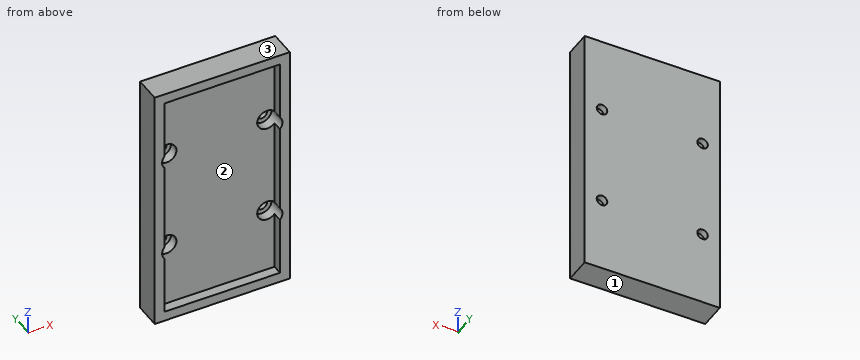
from build123d import *

# Parameters (mm, degrees)
SKETCH1_W                  = 35
SKETCH1_H                  = 70
BOSS_EXTRUDE1_DEPTH        = 5
EXTRUDE_THIN1_DEPTH        = 5
EXTRUDE_THIN1_DEPTH_BACK   = 3
SKETCH9_W                  = 41
SKETCH9_H                  = 76
SKETCH9_W_2                = 35
SKETCH9_H_2                = 70
F_3_2_3_2_DIAMETER_HOLE1_D = 3.2
CUT_EXTRUDE1_DEPTH         = 44.465503563
CUT_EXTRUDE1_DEPTH_BACK    = 3
SKETCH8_R                  = 3


with BuildPart() as part:
    # Sketch1 → Boss-Extrude1 (new body)
    with BuildSketch(Plane(origin=(0, 0, 0), x_dir=(1, 0, 0), z_dir=(0, 1, 0))):
        Rectangle(SKETCH1_W, SKETCH1_H)
    extrude(amount=-BOSS_EXTRUDE1_DEPTH)

    # Sketch9 → Extrude-Thin1 (add, two sides: drawn at the far end of the back side and taken through both)
    with BuildSketch(Plane(origin=(0, -5, 0), x_dir=(1, 0, 0), z_dir=(0, 1, 0)).offset(-EXTRUDE_THIN1_DEPTH_BACK)):
        Rectangle(SKETCH9_W, SKETCH9_H)
        Rectangle(SKETCH9_W_2, SKETCH9_H_2, mode=Mode.SUBTRACT)
    extrude(amount=EXTRUDE_THIN1_DEPTH + EXTRUDE_THIN1_DEPTH_BACK)

    # Ø3.2 (3.2) Diameter Hole1 (through all)
    with Locations(Plane(origin=(0, -5, 0), x_dir=(-1, 0, 0), z_dir=(0, -1, 0))):
        with Locations((15.25, 15.25), (15.25, -15.25), (-15.25, -15.25), (-15.25, 15.25)):
            Hole(F_3_2_3_2_DIAMETER_HOLE1_D / 2)

    # Sketch8 → Cut-Extrude1 (cut, two sides: drawn at the far end of the back side and taken through both)
    with BuildSketch(Plane.XZ.offset(5).offset(-CUT_EXTRUDE1_DEPTH_BACK)):
        with Locations(Location((-15.25, 15.25, 0), (0, 0, 138.590377891))):
            Circle(SKETCH8_R)
        with Locations(Location((15.25, 15.25, 0), (0, 0, 41.409622109))):
            Circle(SKETCH8_R)
        with Locations(Location((15.25, -15.25, 0), (0, 0, 41.409622109))):
            Circle(SKETCH8_R)
        with Locations(Location((-15.25, -15.25, 0), (0, 0, 138.590377891))):
            Circle(SKETCH8_R)
    extrude(amount=CUT_EXTRUDE1_DEPTH + CUT_EXTRUDE1_DEPTH_BACK, mode=Mode.SUBTRACT)


solid = part.part
Geometry check sheet. Reference: the model listing, model coordinates, mm. Face numbers are marked on the shaded views. Round coordinates to 2 decimals unless told otherwise and drop trailing zeros. Loops run counter-clockwise (first coordinate to the right, second up) from the corner with the lowest first, then second, coordinate; pieces in that order, holes last.
Item 1: Cross-section at C-C on y = -3.25. Record the boundary of the cut face in (x, z).
Item 2: Gauge pin test, flat end, axial feed: pin 1 (3.5 mm diameter, centred on x = -15.25, z = -15.25, fed in from -Y). Record the tip position at first contact, or that the pin passes through.
Item 3: Mould release check, pull along Z, two halves, no side actions. Record for the marked faces 1, 2 and 3: pulls with the +Z half, pulls with the -Z half, needs draft (parallel to the pull), parting line crosses it, or undercut.
Item 4: Cross-section at B-B on z = 15.25. Record the boundary of the cut face in (x, y), then the cut area to 3 significant figures.
Item 5: Thickness scan on line 1 (Z direction, x = -15.25, y = -1.2); line 2 (Z direction, x = -17.5, y = -2.25); line 3 (Z direction, x = -6, y = -7). Record the ranges inside material, lowest first.
Item 6: Cross-section at A-A on x = 15.25. Record the boundary of the cut face in (y, z), then the cut area to 3 significant figures.
Item 7: Cross-section at D-D on x = 6. Record the boundary of the cut face in (y, z).
Answer sheet:
1. outline: (-20.5, -38) - (20.5, -38) - (20.5, 38) - (-20.5, 38) - close; hole circle Ø6 at (-15.25, -15.25); hole circle Ø6 at (-15.25, 15.25); hole circle Ø6 at (15.25, -15.25); hole circle Ø6 at (15.25, 15.25)
2. pin 1: stops at y = -2
3. face 1: pulls with the -Z half
3. face 2: undercut
3. face 3: pulls with the +Z half
4. outline: (-20.5, -8) - (-18.25, -8) - (-18.25, -2) - (-16.85, -2) - (-16.85, 0) - (-20.5, 0) - close; (-13.65, -2) - (-12.25, -2) - (-12.25, -5) - (12.25, -5) - (12.25, -2) - (13.65, -2) - (13.65, 0) - (-13.65, 0) - close; (16.85, -2) - (18.25, -2) - (18.25, -8) - (20.5, -8) - (20.5, 0) - (16.85, 0) - close
4. area: 170 mm2
5. line 1: z = -38 to -16.85, -13.65 to 13.65, 16.85 to 38
5. line 2: z = -38 to -17.23, -13.27 to 13.27, 17.23 to 38
5. line 3: z = -38 to -35, 35 to 38
6. outline: (-8, -38) - (0, -38) - (0, -16.85) - (-2, -16.85) - (-2, -18.25) - (-5, -18.25) - (-5, -35) - (-8, -35) - close; (-8, 35) - (-5, 35) - (-5, 18.25) - (-2, 18.25) - (-2, 16.85) - (0, 16.85) - (0, 38) - (-8, 38) - close; (-5, -12.25) - (-2, -12.25) - (-2, -13.65) - (0, -13.65) - (0, 13.65) - (-2, 13.65) - (-2, 12.25) - (-5, 12.25) - close
6. area: 349 mm2
7. outline: (-8, -38) - (0, -38) - (0, 38) - (-8, 38) - (-8, 35) - (-5, 35) - (-5, -35) - (-8, -35) - close
